The model under review builds one solid part; all positions refer to its coordinate system, in mm. A direction names the side the tool comes from. Give positions to 0.01 mm unless a question says otherwise; leave off trailing zeros. Order: outer loops, then holes, each group sorted by start corner. A loop starts at its lowest first (then second) coordinate and runs counter-clockwise, first axis right, second up. Notation, with made-up numbers: (-15.75, 3.5) - (11.25, 3.5) arc R6 ccw to (11.25, 13.5) - close; hole circle Ø5 at (-13.5, 81). An arc over 180 degrees is marked (long way). Use CSV: the item, a comma, the result in double quotes. Start each with the question number.
```python
from build123d import *

# Parameters (mm, degrees)
SKETCH2_W           = 500
SKETCH2_H           = 40
BOSS_EXTRUDE1_DEPTH = 40
SKETCH3_W           = 38
SKETCH3_H           = 38
CUT_EXTRUDE1_DEPTH  = 500
CUT_EXTRUDE2_DEPTH  = 10


with BuildPart() as part:
    # Sketch2 → Boss-Extrude1 (new body)
    with BuildSketch(Plane.XY):
        with Locations((-79.545454545, 73.276515152)):
            Rectangle(SKETCH2_W, SKETCH2_H)
    extrude(amount=BOSS_EXTRUDE1_DEPTH)

    # Sketch3 → Cut-Extrude1 (cut)
    with BuildSketch(Plane.ZY.offset(329.545454545)):
        with Locations((21, 72.276515152)):
            Rectangle(SKETCH3_W, SKETCH3_H)
    extrude(amount=-CUT_EXTRUDE1_DEPTH, mode=Mode.SUBTRACT)

    # Sketch4 → Cut-Extrude2 (cut)
    with BuildSketch(Plane(origin=(0, 93.276515152, 0), x_dir=(1, 0, 0), z_dir=(0, 1, 0))):
        Polygon((-329.545454545, 0), (-329.545454545, -40), (-289.545454545, -40), align=None)
        Polygon((170.454545455, -40), (170.454545455, 0), (130.454545455, -40), align=None)
    extrude(amount=-CUT_EXTRUDE2_DEPTH, mode=Mode.SUBTRACT)


solid = part.part
```
1. To check wall thickness, follow L1, parallel to Y at x = -37.5, z = 25; L2, parallel to Z at x = -181, y = 84. State the ranges of each line that lie inside material, in increasing order. Write a range as [from, to].
2. Consider section A-A (x = -150). Give the boundary of the cut face in (y, z), and give its area (3 significant figures).
3. Consider section C-C (z = 18). Give the boundary of the cut face in (x, y), and give its area (3 significant figures).
4. Tool access review of faces 1 (the face through (-83, 93.277, 20)), 2 (the face through (-83, 74, 0)), 3 (the face through (-312.415, 91.633, 17.13)), 4 (the face through (-83, 72, 2)), 5 (the face through (153.511, 91.633, 16.944)): name each direction out of +Z, -Z, +X, -X, +Y, -Y from which nothing blocks a thin tool from reaching the whole face with its end or side.
5. Clearance check with flat-ended pins moving along their axes: pin 1 (12 mm diameter, centred on y = 89, z = 34.5, fed in from +X); pin 2 (8 mm diameter, centred on x = 102.5, y = 61.5, fed in from +Z); pin 3 (19 mm diameter, centred on x = -60, z = 19.5, fed in from -Y). State where each tip first meets the part, or that it passes through.
6. Consider section B-B (y = 78.5). Give the boundary of the cut face in (x, z), and give its area (3 significant figures).
Answers follow:
1,L1,"y = [91.28, 93.28]"
1,L2,"z = [0, 2]"
2,outline,"(53.28, 0) - (93.28, 0) - (93.28, 40) - (91.28, 40) - (91.28, 2) - (53.28, 2) - close"
2,area,"156 mm^2"
3,outline,"(-311.55, 91.28) - (152.45, 91.28) - (152.45, 93.28) - (-311.55, 93.28) - close"
3,area,"928 mm^2"
4,face 1,"+Z, -Z, +X, -X, +Y"
4,face 2,"-Z, +X, -X, +Y, -Y"
4,face 3,"+Z, -X, +Y"
4,face 4,"+Z, +X, -X, -Y"
4,face 5,"+Z, +X, +Y"
5,pin 1,"stops at x = 141.51"
5,pin 2,"stops at z = 2"
5,pin 3,"stops at y = 91.28"
6,outline,"(-329.55, 0) - (170.45, 0) - (170.45, 2) - (-329.55, 2) - close"
6,area,"1,000 mm^2"
